The model under review builds one solid part; all positions refer to its coordinate system, in mm. A direction names the side the tool comes from. Give positions to 0.01 mm unless a question says otherwise; leave off trailing zeros. Order: outer loops, then holes, each group sorted by start corner. A loop starts at its lowest first (then second) coordinate and runs counter-clockwise, first axis right, second up. Notation, with made-up numbers: (69, 39.5) -> (83, 39.5) arc R25 cw to (83, 73.5) -> close; hole circle Ø6 at (78, 68.5). An arc over 180 degrees is marked (long way). Use one line per item in the form item = value.
```python
from build123d import *

# Parameters (mm, degrees)
F0_W     = 102
F0_H     = 40
F1_DEPTH = 3
F2_W     = 3
F2_H     = 5
F3_DEPTH = 3
F4_W     = 5
F4_H     = 3
F5_DEPTH = 3
F6_W     = 114.49237
F6_H     = 23.447346
F7_DEPTH = 25
F8_W     = 3
F8_H     = 5
F9_DEPTH = 25


with BuildPart() as f1:
    # F0 (on Front) → F1 (new body)
    with BuildSketch(Plane.XZ):
        Rectangle(F0_W, F0_H)
    extrude(amount=F1_DEPTH)

    # F2 (on face) → F3 (join)
    with BuildSketch(Plane.XZ.offset(3)):
        with Locations((-52.5, -17.5)):
            Rectangle(F2_W, F2_H)
        with Locations((-52.5, -7.5)):
            Rectangle(F2_W, F2_H)
        with Locations((-52.5, 2.5)):
            Rectangle(F2_W, F2_H)
        with Locations((-52.5, 12.5)):
            Rectangle(F2_W, F2_H)
        with Locations((52.5, -7.5)):
            Rectangle(F2_W, F2_H)
        with Locations((52.5, -17.5)):
            Rectangle(F2_W, F2_H)
        with Locations((52.5, 12.5)):
            Rectangle(F2_W, F2_H)
        with Locations((52.5, 2.5)):
            Rectangle(F2_W, F2_H)
    extrude(amount=-F3_DEPTH)

    # F4 (on face) → F5 (join)
    with BuildSketch(Plane.XZ.offset(3)):
        with Locations((5, -21.5)):
            Rectangle(F4_W, F4_H)
        with Locations((15, -21.5)):
            Rectangle(F4_W, F4_H)
        with Locations((25, -21.5)):
            Rectangle(F4_W, F4_H)
        with Locations((35, -21.5)):
            Rectangle(F4_W, F4_H)
        with Locations((45, -21.5)):
            Rectangle(F4_W, F4_H)
        with Locations((-25, -21.5)):
            Rectangle(F4_W, F4_H)
        with Locations((-15, -21.5)):
            Rectangle(F4_W, F4_H)
        with Locations((-5, -21.5)):
            Rectangle(F4_W, F4_H)
        with Locations((-35, -21.5)):
            Rectangle(F4_W, F4_H)
        with Locations((-45, -21.5)):
            Rectangle(F4_W, F4_H)
    extrude(amount=-F5_DEPTH)

    # F6 (on face) → F7 (cut)
    with BuildSketch(Plane.XZ.offset(3)):
        with Locations((3.246185, 11.723673)):
            Rectangle(F6_W, F6_H)
    extrude(amount=-F7_DEPTH, mode=Mode.SUBTRACT)

    # F8 (on face) → F9 (cut)
    with BuildSketch(Plane(origin=(0, 0, 0), x_dir=(-1, 0, 0), z_dir=(0, 1, 0))):
        with Locations((-35, -17.5)):
            Rectangle(F8_W, F8_H)
        with Locations((-35, -7.5)):
            Rectangle(F8_W, F8_H)
        with Locations((35, -7.5)):
            Rectangle(F8_W, F8_H)
        with Locations((35, -17.5)):
            Rectangle(F8_W, F8_H)
    extrude(amount=-F9_DEPTH, mode=Mode.SUBTRACT)


solid = f1.part
```
1. Add section C-C on z = -21.5. Count the separate pieces of the cut face and the enclosed holes in it, then the cut area to 3 significant figures.
Values:
separate_pieces = 10
enclosed_holes = 0
area = 150 mm^2
2. Tool access review of faces 1 (the face through (-35, -1, -10)), 2 (the face through (-53, -2, -5)), 3 (the face through (32.5, -2, -22)): name each direction out of +Z, -Z, +X, -X, +Y, -Y from which nothing blocks a thin tool from reaching the whole face with its end or side.
Values:
face_1 = +Y, -Y
face_2 = +Z, -X, +Y, -Y
face_3 = -Z, +Y, -Y
3. For pin 1 Ø1.5 at (y, z) = (-2, -21.5) entering from -X, flat-tipped, find the tip position at first contact; note if it passes through.
Values:
pin_1 = -47.5
4. For L1, parallel to X at y = -2.35, z = -7.75; L2, parallel to X at y = -2.5, z = -3; L3, parallel to Z at x = 9, y = -2.55, list the stretches that pass through material, from the lowest coordinate up.
Values:
L1 = -54 to -36.5, -33.5 to 33.5, 36.5 to 54
L2 = -51 to 51
L3 = -20 to 0
5. The part is to be moulded in two halves that separate along X. For faces 4 (the face through (37.5, -2, -22)), 5 (the face through (-1, -3, -11)), 6 (the face through (-54, -2, -18)), 7 (the face through (7.5, -2, -22)), say which applies: +X half, -X half, draft (parallel to the pull), parting line (faces both ways), or undercut.
Values:
face_4 = undercut
face_5 = draft
face_6 = -X half
face_7 = undercut
6. Add section B-B on z = -17.5. Give the boundary of the cut face in (x, y).
Values:
outline = (-54, -3) -> (-36.5, -3) -> (-36.5, 0) -> (-54, 0) -> close; (-33.5, -3) -> (33.5, -3) -> (33.5, 0) -> (-33.5, 0) -> close; (36.5, -3) -> (54, -3) -> (54, 0) -> (36.5, 0) -> close
7. Add section A-A on x = -35.5. Give the boundary of the cut face in (y, z), then the cut area to 3 significant figures.
Values:
outline = (-3, -23) -> (0, -23) -> (0, -20) -> (-3, -20) -> close; (-3, -15) -> (0, -15) -> (0, -10) -> (-3, -10) -> close; (-3, -5) -> (0, -5) -> (0, 0) -> (-3, 0) -> close
area = 39.0 mm^2
